from build123d import *

# Parameters (mm, degrees)
F0_R          = 8.763
F1_DEPTH      = 59.436
F1_DEPTH_BACK = 59.436
F2_R          = 3.556
F3_DEPTH      = 76.2
F3_DEPTH_BACK = 76.2
F6_R          = 8.763
F7_DEPTH      = 11.684
F8_R          = 8.763
F9_DEPTH      = 11.684


with BuildPart() as f1:
    # F0 (on Top) → F1 (new body, two sides)
    with BuildSketch(Plane.XY) as f1_sk:
        Circle(F0_R)
    extrude(amount=F1_DEPTH)
    extrude(f1_sk.sketch, amount=-F1_DEPTH_BACK)

    # F2 (on Top) → F3 (join, two sides)
    with BuildSketch(Plane.XY) as f3_sk:
        Circle(F2_R)
    extrude(amount=F3_DEPTH)
    extrude(f3_sk.sketch, amount=-F3_DEPTH_BACK)

    # F6 (on offset) → F7 (join)
    with BuildSketch(Plane.XY.offset(76.2)):
        Circle(F6_R)
    extrude(amount=-F7_DEPTH)

    # F8 (on offset) → F9 (join)
    with BuildSketch(Plane.XY.offset(-76.2)):
        Circle(F8_R)
    extrude(amount=F9_DEPTH)


solid = f1.part
Can you work these out from the model? Positions are in its coordinate system, mm. A direction names the side the tool comes from. Coordinates: 2 decimals unless noted, no trailing zeros. Order: outer loops, then holes, each group sorted by start corner. A loop starts at its lowest first (then second) coordinate and runs counter-clockwise, first axis right, second up. Notation, with made-up numbers: (78.25, -29) -> (85.25, -29) arc R21 ccw to (85.25, -1) -> close; hole circle Ø11 at (4.5, 52.25). An arc over 180 degrees is marked (long way). Use one line per item in the form item = value.
Q1. Imagine slicing it at C-C, the plane y = 0. List the corners of the cut face in (x, z) for me, then the cut area to 3 significant figures.
From the geometry:
outline = (-8.76, -76.2) -> (8.76, -76.2) -> (8.76, -64.52) -> (3.56, -64.52) -> (3.56, -59.44) -> (8.76, -59.44) -> (8.76, 59.44) -> (3.56, 59.44) -> (3.56, 64.52) -> (8.76, 64.52) -> (8.76, 76.2) -> (-8.76, 76.2) -> (-8.76, 64.52) -> (-3.56, 64.52) -> (-3.56, 59.44) -> (-8.76, 59.44) -> (-8.76, -59.44) -> (-3.56, -59.44) -> (-3.56, -64.52) -> (-8.76, -64.52) -> close
area = 2,570 mm²
Q2. We'd pull the mould along Z, two halves only. Please class faces 1 (the face through (0, 0, -76.2)), 2 (the face through (8.36, 2.63, 70.44)), 3 (the face through (0, 0, 76.2)), 4 (the face through (-0.77, -3.47, 61.94)): released by +Z, released by -Z, zero draft, split by the parting line, or undercut.
From the geometry:
face_1 = released by -Z
face_2 = zero draft
face_3 = released by +Z
face_4 = undercut
Q3. Imagine slicing it at B-B, the plane x = -5.25. List the corners of the cut face in (y, z) for me, then the cut area to 3 significant figures.
From the geometry:
outline = (-7.02, -76.2) -> (7.02, -76.2) -> (7.02, -64.52) -> (-7.02, -64.52) -> close; (-7.02, -59.44) -> (7.02, -59.44) -> (7.02, 59.44) -> (-7.02, 59.44) -> close; (-7.02, 64.52) -> (7.02, 64.52) -> (7.02, 76.2) -> (-7.02, 76.2) -> close
area = 2,000 mm²
Q4. Will these pins go through, and if not, where does the flat tip stop? P1, Ø2, axis at y = -4, z = -9.5, coming from the +X side; P2, Ø6, axis at x = 4.5, z = 26, coming from the +Y side; P3, Ø4, axis at x = -1.5, z = -39, coming from the +Y side.
From the geometry:
P1 = 8.23
P2 = 8.63
P3 = 8.76
Q5. Imagine slicing it at A-A, the plane y = 6.5. List the corners of the cut face in (x, z) for me.
From the geometry:
outline = (-5.88, -76.2) -> (5.88, -76.2) -> (5.88, -64.52) -> (-5.88, -64.52) -> close; (-5.88, -59.44) -> (5.88, -59.44) -> (5.88, 59.44) -> (-5.88, 59.44) -> close; (-5.88, 64.52) -> (5.88, 64.52) -> (5.88, 76.2) -> (-5.88, 76.2) -> close
Q6. Imagine slicing it at D-D, the plane z = 46. List the corners of the cut face in (x, y) for me.
From the geometry:
outline = circle Ø17.53 at (0, 0)
Q7. Which directions (+Z, -Z, +X, -X, +Y, -Y) give clear straight access to the entire face, cutting with the end or side of a thin tool? Please do faces 5 (the face through (4, 0, 59.436)), 6 (the face through (8.36, 2.63, -70.44)).
From the geometry:
face_5 = none
face_6 = +Z, -Z
Q8. I need wall thicknesses on L1, parallel to Z at x = -4.25, y = -3.75; L2, parallel to Y at x = 8, z = -48; L3, parallel to Y at x = 1.75, z = -34. Which ranges of each line are inside material? Lowest first, please.
From the geometry:
L1 = -76.2 to -64.52, -59.44 to 59.44, 64.52 to 76.2
L2 = -3.58 to 3.58
L3 = -8.59 to 8.59
